Check sheet for the drawn part. Datum: minimum x, y, z corner. Units: mm. Give positions to 0.01 mm unless a question says otherwise; leave off trailing zeros. Order: outer loops, then holes, each group sorted by start corner. A loop starts at its lowest first (then second) coordinate and runs counter-clockwise, first axis right, second up. Notation, with made-up numbers: (-33.75, -34.75) - (3.25, -34.75) arc R7 cw to (3.25, -25.75) - close; hole circle Ø9 at (58.5, -31). An arc over 180 degrees is marked (long way). Answer as a JSON object with one key per item and string values. Group by question number.
(1) Section check B-B (x = 1.5). Count the separate pieces of the cut face and the enclosed holes in it, then the cut area to 3 significant figures.
(2) Thickness scan on line 1 (Y direction, x = 3, z = 91.6); line 2 (Y direction, x = 3, z = 50); line 3 (Z direction, x = 1.5, y = 49.5). Record the ranges inside material, lowest first.
(3) Section check A-A (z = 91.6). Record the boundary of the cut face in (x, y).
(4) Section check C-C (y = 10). Record the boundary of the cut face in (x, z), then the cut area to 3 significant figures.
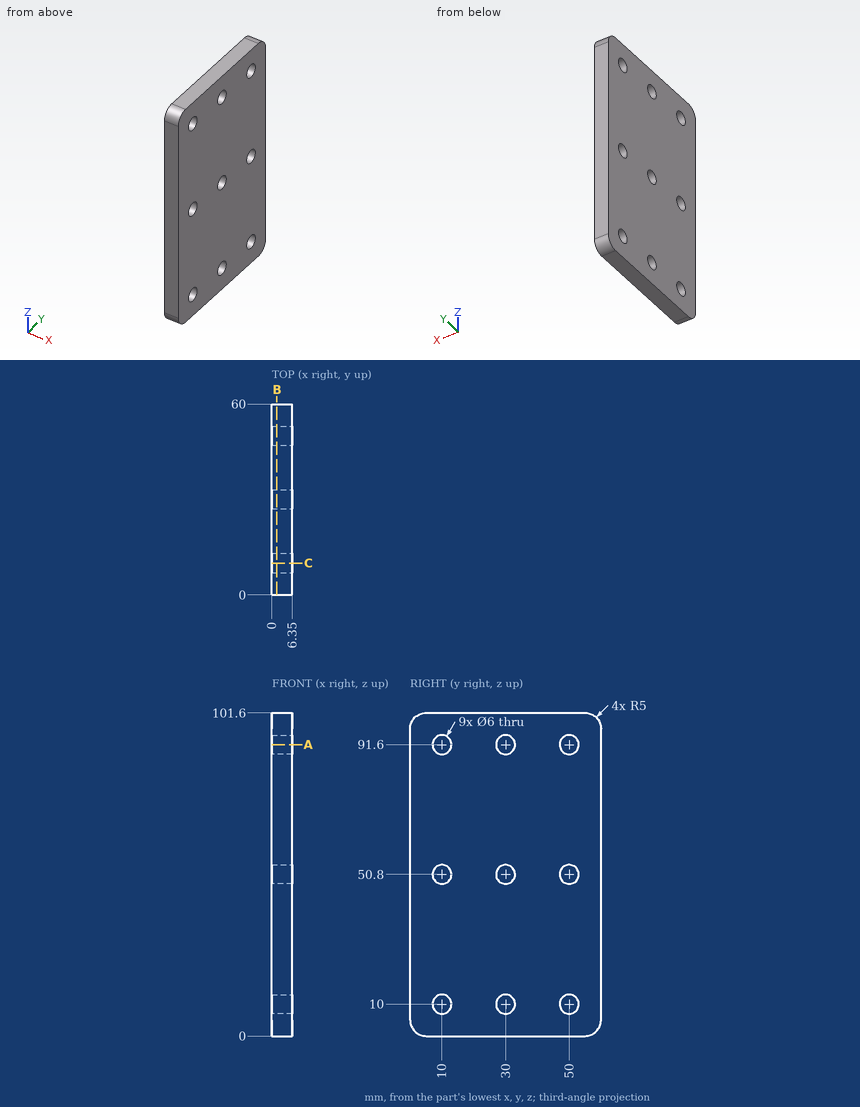
Solutions:
{
 "1": {"separate pieces": "1", "enclosed holes": "9", "area": "5,820 mm2"},
 "2": {"line 1": "y = 0 to 7, 13 to 27, 33 to 47, 53 to 60", "line 2": "y = 0 to 7.11, 12.89 to 27.11, 32.89 to 47.11, 52.89 to 60", "line 3": "z = 0 to 7.04, 12.96 to 47.84, 53.76 to 88.64, 94.56 to 101.6"},
 "3": {"outline": "(0, 0) - (6.35, 0) - (6.35, 7) - (0, 7) - close; (0, 13) - (6.35, 13) - (6.35, 27) - (0, 27) - close; (0, 33) - (6.35, 33) - (6.35, 47) - (0, 47) - close; (0, 53) - (6.35, 53) - (6.35, 60) - (0, 60) - close"},
 "4": {"outline": "(0, 0) - (6.35, 0) - (6.35, 7) - (0, 7) - close; (0, 13) - (6.35, 13) - (6.35, 47.8) - (0, 47.8) - close; (0, 53.8) - (6.35, 53.8) - (6.35, 88.6) - (0, 88.6) - close; (0, 94.6) - (6.35, 94.6) - (6.35, 101.6) - (0, 101.6) - close", "area": "531 mm2"}
}
